Here's how the part is built. I have some questions about the finished solid (model axes, mm). Face numbers are marked on the shaded views. Coordinates: 2 decimals unless noted, no trailing zeros. Write each loop counter-clockwise with the first axis right and the second up, starting at its lowest first coordinate (ties: lowest second). Pieces come first, ordered by that corner, then holes.
Item 1: We'd pull the mould along Z, two halves only. Please class the marked faces 1 and 2: +Z half, -Z half, draft (parallel to the pull), parting line (faces both ways), or undercut.
Item 2: If we section it at B-B (x = 0): Count the separate pieces of the cut face and the enclosed holes in it, then the cut area to 3 significant figures.
Item 3: If we section it at D-D (y = 23.5): Please give me the cut outline in (x, z).
Item 4: If we section it at C-C (y = 48): Please give me the cut outline in (x, z), then the cut area to 3 significant figures.
Item 5: I'm going to push flat-ended pins straight in: pin 1 Ø5 at (x, z) = (-52.5, -31.5) entering from +Y; pin 2 Ø10 at (x, z) = (43, -74) entering from -Y; pin 3 Ø12 at (x, z) = (-46.5, 14) entering from +Y. Where does each tip first touch, or does it pass through?
Item 6: If I drill on line 1 (X direction, y = 12, z = 0); line 2 (Z direction, x = 0, y = 14); line 3 (X direction, y = 107, z = 79), over which ranges is the centre line in solid material (lowest first)?
from build123d import *
from build123d.topology import SkipClean

# Parameters (mm, degrees)
SKETCH3_R          = 20.5
CUT_EXTRUDE1_DEPTH = 2.5


with BuildPart() as part:
    # Sketch2 → Revolve1 (revolve)
    with BuildSketch(Plane.XY, mode=Mode.PRIVATE) as revolve1_sk:
        with BuildLine():
            Line((-12, 0), (-10.5, 0))
            Line((-10.5, 0), (-10.5, 30))
            ThreePointArc((-10.5, 30), (-10.728361402, 31.148050297), (-11.378679656, 32.121320344))
            Line((-11.378679656, 32.121320344), (-99.257359313, 120))
            Line((-99.257359313, 120), (-101.378679656, 120))
            Line((-101.378679656, 120), (-12.43972081, 31.061041153))
            Line((-12.43972081, 31.061041153), (-12.439339828, 31.060660172))
            ThreePointArc((-12.439339828, 31.060660172), (-12.114180701, 30.574025149), (-12, 30))
            Line((-12, 30), (-12, 0))
        make_face()
    revolve(revolve1_sk.sketch.rotate(Axis((0, 0, 0), (0, 1, 0)), 270), axis=Axis((0, 0, 0), (0, 1, 0)))

    # Sketch3 → Cut-Extrude1 (cut, symmetric)
    with SkipClean():  # the faces are left unmerged after this step: merging them gives an invalid solid
        with BuildSketch(Plane(origin=(0, 0, 0), x_dir=(0, 0, -1), z_dir=(1, 0, 0))):
            with Locations((25, 20)):
                Circle(SKETCH3_R)
        extrude(amount=CUT_EXTRUDE1_DEPTH, both=True, mode=Mode.SUBTRACT)


solid = part.part
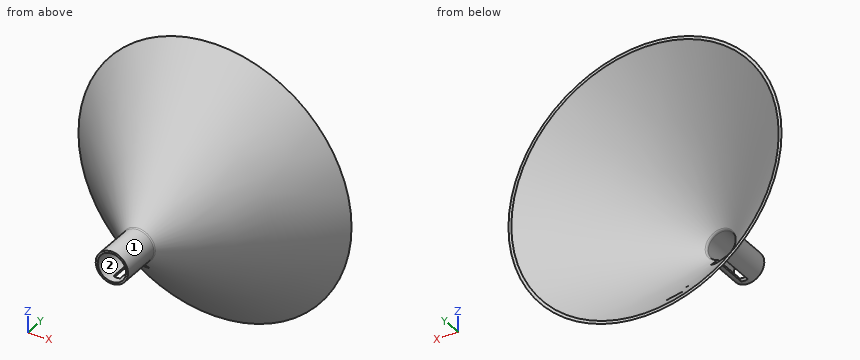
Answer list:
1. face 1: parting line
1. face 2: undercut
2. separate pieces: 3
2. enclosed holes: 0
2. area: 412 mm2
3. outline: (-2.5, -11.74) - (-2.5, -10.2) arc R10.5 cw (long way) to (2.5, -10.2) - (2.5, -11.74) arc R12 ccw (long way) to start
4. outline: circle Ø58.76 at (0, 0); hole circle Ø54.51 at (0, 0)
4. area: 377 mm2
5. pin 1: stops at y = 84.47
5. pin 2: stops at y = 99.21
5. pin 3: stops at y = 75.3
6. line 1: x = -12 to -10.5, 10.5 to 12
6. line 2: z = 10.5 to 12
6. line 3: x = -39.62 to -34.63, 34.63 to 39.62
